Read the model definition and answer for the solid it produces. Units are mm, in the model's axes. A direction names the side the tool comes from. Coordinates: 2 decimals unless noted, no trailing zeros. Write each loop counter-clockwise with the first axis right and the second up, starting at its lowest first coordinate (ties: lowest second). Pieces come first, ordered by that corner, then holes.
from build123d import *

# Parameters (mm, degrees)
SKETCH1_R             = 20
SKETCH1_R_2           = 7.5
BOSS_EXTRUDE1_DEPTH   = 17
BOSS_EXTRUDE1_2_DEPTH = 17
SKETCH1_R_3           = 25
SKETCH1_R_4           = 8
BOSS_EXTRUDE1_3_DEPTH = 17
BOSS_EXTRUDE4_DEPTH   = 15
SKETCH1_12_R          = 3
BOSS_EXTRUDE5_DEPTH   = 6


with BuildPart() as part:
    # Sketch1 → Boss-Extrude1 (new body)
    with BuildSketch(Plane(origin=(0, 0, 0), x_dir=(1, 0, 0), z_dir=(0, 1, 0))):
        with Locations(Location((-75, 175, 0), (0, 0, 270))):
            Circle(SKETCH1_R)
        with Locations(Location((-75, 175, 0), (0, 0, 270))):
            Circle(SKETCH1_R_2, mode=Mode.SUBTRACT)
    extrude(amount=BOSS_EXTRUDE1_DEPTH)



with BuildPart() as body_2:
    # Sketch1 → Boss-Extrude1 2 (new body)
    with BuildSketch(Plane(origin=(0, 0, 0), x_dir=(1, 0, 0), z_dir=(0, 1, 0))):
        with Locations(Location((75, 175, 0), (0, 0, 270))):
            Circle(SKETCH1_R)
        with Locations(Location((75, 175, 0), (0, 0, 270))):
            Circle(SKETCH1_R_2, mode=Mode.SUBTRACT)
    extrude(amount=BOSS_EXTRUDE1_2_DEPTH)


with BuildPart() as body_3:
    # Sketch1 → Boss-Extrude1 3 (new body)
    with BuildSketch(Plane(origin=(0, 0, 0), x_dir=(1, 0, 0), z_dir=(0, 1, 0))):
        with Locations(Location((0, 0, 0), (0, 0, 270))):
            Circle(SKETCH1_R_3)
        with Locations(Location((0, 0, 0), (0, 0, 270))):
            Circle(SKETCH1_R_4, mode=Mode.SUBTRACT)
    extrude(amount=BOSS_EXTRUDE1_3_DEPTH)


with BuildPart() as part_1:
    add(part.part)

    add(body_2.part)  # Boss-Extrude4 merges body 2

    add(body_3.part)  # Boss-Extrude4 merges body 3
    # Sketch1_11 → Boss-Extrude4 (add)
    with BuildSketch(Plane(origin=(0, 0, 0), x_dir=(1, 0, 0), z_dir=(0, 1, 0))):
        with BuildLine():
            Line((-37.860985847, 80.673340544), (-77.990381057, 150.179491924))
            ThreePointArc((-77.990381057, 150.179491924), (-65.179491924, 152.009618943), (-55, 160))
            Line((-55, 160), (55, 160))
            ThreePointArc((55, 160), (65.179491924, 152.009618943), (77.990381057, 150.179491924))
            Line((77.990381057, 150.179491924), (37.860985847, 80.673340544))
            ThreePointArc((37.860985847, 80.673340544), (26.459547, 48.078091436), (20.690948252, 14.031559444))
            ThreePointArc((20.690948252, 14.031559444), (23.898469682, 7.339151643), (25, 0))
            ThreePointArc((25, 0), (29.68582744, 40.076807855), (42.320508076, 78.397459622))
            Line((42.320508076, 78.397459622), (92.320508076, 165))
            ThreePointArc((92.320508076, 165), (69.823619098, 155.681483474), (55, 175))
            ThreePointArc((55, 175), (52.071067812, 167.928932188), (45, 165))
            Line((45, 165), (0, 165))
            Line((0, 165), (-45, 165))
            ThreePointArc((-45, 165), (-52.071067812, 167.928932188), (-55, 175))
            ThreePointArc((-55, 175), (-69.823619098, 155.681483474), (-92.320508076, 165))
            Line((-92.320508076, 165), (-42.320508076, 78.397459622))
            ThreePointArc((-42.320508076, 78.397459622), (-29.68582744, 40.076807855), (-25, 0))
            ThreePointArc((-25, 0), (-23.898469682, 7.339151643), (-20.690948252, 14.031559444))
            ThreePointArc((-20.690948252, 14.031559444), (-26.459547, 48.078091436), (-37.860985847, 80.673340544))
        make_face()
    extrude(amount=BOSS_EXTRUDE4_DEPTH)

    # Sketch1_12 → Boss-Extrude5 (add)
    with BuildSketch(Plane(origin=(0, 0, 0), x_dir=(1, 0, 0), z_dir=(0, 1, 0))):
        with BuildLine():
            ThreePointArc((-55, 160), (-65.179491924, 152.009618943), (-77.990381057, 150.179491924))
            Line((-77.990381057, 150.179491924), (-37.860985847, 80.673340544))
            ThreePointArc((-37.860985847, 80.673340544), (-26.459547, 48.078091436), (-20.690948252, 14.031559444))
            ThreePointArc((-20.690948252, 14.031559444), (0, 25), (20.690948252, 14.031559444))
            ThreePointArc((20.690948252, 14.031559444), (26.459547, 48.078091436), (37.860985847, 80.673340544))
            Line((37.860985847, 80.673340544), (77.990381057, 150.179491924))
            ThreePointArc((77.990381057, 150.179491924), (65.179491924, 152.009618943), (55, 160))
            Line((55, 160), (-55, 160))
        make_face()
        with BuildLine():
            Line((41.02974036, 124.272968417), (11.02974036, 54.272968417))
            ThreePointArc((11.02974036, 54.272968417), (0, 47), (-11.02974036, 54.272968417))
            Line((-11.02974036, 54.272968417), (-41.02974036, 124.272968417))
            ThreePointArc((-41.02974036, 124.272968417), (-33.939530359, 140.334906288), (-18.416073702, 132.132515207))
            Line((-18.416073702, 132.132515207), (-11.583926298, 106.867484793))
            ThreePointArc((-11.583926298, 106.867484793), (0, 98), (11.583926298, 106.867484793))
            Line((11.583926298, 106.867484793), (18.416073702, 132.132515207))
            ThreePointArc((18.416073702, 132.132515207), (33.939530359, 140.334906288), (41.02974036, 124.272968417))
        make_face(mode=Mode.SUBTRACT)
        with Locations(Location((0, 110, 0), (0, 0, 270))):
            Circle(SKETCH1_12_R, mode=Mode.SUBTRACT)
    extrude(amount=BOSS_EXTRUDE5_DEPTH)


solid = part_1.part
Item 1: Find the intervals of material crossed by probe 1 along X at (y, z) = (5.25, -175); probe 2 along Z at (x, y) = (69.5, 9.25); probe 3 along Z at (x, y) = (74, 6.25), in increasing order.
Item 2: The part is cut by section D-D (x = -75). Give the vertices of the cut face in (y, z), and give its area (3 significant figures).
Item 3: The part is cut by section C-C (z = -121). Give the vertices of the cut face in (x, y).
Item 4: For faces 1 (the cylindrical face through (-34.2, 2.96, -140.24)), 2 (the cylindrical face through (52.15, 7.4, -168.01)), 3 (the flat face through (-57.645, 10.437, -114.94)), determine the directions among +Z, -Z, +X, -X, +Y, -Y from which every point of the face is accessible in a straight line to the end or side of a thin tool.
Item 5: Given pin 1 (1 mm diameter, centred on y = 15, z = -47.5, fed in from -X); pin 2 (1.5 mm diameter, centred on y = 12.5, z = -113, fed in from -X); pin 3 (9.5 mm diameter, centred on x = 0, z = -110, fed in from -Y); pin 4 (2 mm diameter, centred on y = 10.5, z = -90, fed in from +X), each flat-ended and moving along its own axis, determine where each tip first touches the part or whether it passes through.
Item 6: The part is cut by section A-A (y = 2.5). Give the vertices of the cut face in (x, z).
Item 7: Determine the mould class of faces 4 (the flat face through (66.97, 7.4, -121.09)), 5 (the cylindrical face through (72.13, 8.38, -168.07)), 6 (the cylindrical face through (33.68, 2.96, -140.42)), 7 (the flat face through (75, 17, -166)) for opening direction X: +X half, -X half, draft (parallel to the pull), parting line (faces both ways), or undercut.
Item 8: The part is cut by section B-B (x = 0). Give the vertices of the cut face in (y, z), and give its area (3 significant figures).
Answer:
1. probe 1: x = -95 to -82.5, -67.5 to -55, 55 to 67.5, 82.5 to 95
1. probe 2: z = -194.23 to -180.1, -169.9 to -150.61, -135.47 to -125.47
1. probe 3: z = -194.97 to -182.43, -167.57 to -150.02, -143.27 to -133.27
2. outline: (0, -195) - (17, -195) - (17, -182.5) - (0, -182.5) - close; (0, -167.5) - (17, -167.5) - (17, -155) - (15, -155) - (15, -150) - (6, -150) - (6, -145) - (15, -145) - (15, -135) - (0, -135) - close
2. area: 680 mm2
3. outline: (-66.92, 0) - (-39.63, 0) - (-39.63, 6) - (-61.14, 6) - (-61.14, 15) - (-66.92, 15) - close; (-15.41, 0) - (15.41, 0) - (15.41, 6) - (-15.41, 6) - close; (39.63, 0) - (66.92, 0) - (66.92, 15) - (61.14, 15) - (61.14, 6) - (39.63, 6) - close
4. face 1: +Y, -Y
4. face 2: -Z, +Y, -Y
4. face 3: +Y
5. pin 1: stops at x = -31.61
5. pin 2: stops at x = -62.73
5. pin 3: stops at y = 0
5. pin 4: stops at x = 49.6
6. outline: (-92.32, -165) arc R20 ccw (long way) to (-55, -175) arc R10 cw to (-45, -165) - (45, -165) arc R10 cw to (55, -175) arc R20 ccw (long way) to (92.32, -165) - (42.32, -78.4) arc R200 cw to (25, 0) arc R25 ccw to (-25, 0) arc R200 cw to (-42.32, -78.4) - close; hole circle Ø15 at (-75, -175); hole (-41.03, -124.27) arc R12 ccw (long way) to (-18.42, -132.13) - (-11.58, -106.87) arc R12 cw to (11.58, -106.87) - (18.42, -132.13) arc R12 ccw (long way) to (41.03, -124.27) - (11.03, -54.27) arc R12 ccw to (-11.03, -54.27) - close; hole circle Ø16 at (0, 0); hole circle Ø6 at (0, -110); hole circle Ø15 at (75, -175)
7. face 4: +X half
7. face 5: undercut
7. face 6: undercut
7. face 7: draft
8. outline: (0, -165) - (15, -165) - (15, -160) - (6, -160) - (6, -113) - (0, -113) - close; (0, -107) - (6, -107) - (6, -98) - (0, -98) - close; (0, -47) - (6, -47) - (6, -25) - (17, -25) - (17, -8) - (0, -8) - close; (0, 8) - (17, 8) - (17, 25) - (0, 25) - close
8. area: 1,120 mm2
